```python
from build123d import *

# Parameters (mm, degrees)
PAD001_DEPTH        = 35
HOLE002_D           = 5.5
HOLE002_CSINK_D     = 10
HOLE002_CSINK_ANGLE = 90
SKETCH004_R         = 6.501169
SKETCH004_R_2       = 5.481256
POCKET_DEPTH        = 13.6312167212
SKETCH007_W         = 3.5
SKETCH007_H         = 35
POCKET002_DEPTH     = 1
CHAMFER_SIZE        = 0.99
FILLET007_R         = 3
FILLET008_R         = 1


with BuildPart() as part:
    # Sketch002 → Pad001 (new body)
    with BuildSketch(Plane.YZ):
        with BuildLine():
            Line((-188.1964293023, 612.8903873712), (-179.4587343049, 634.2262558534))
            Line((-171.1300961638, 630.8154221261), (-179.4587343049, 634.2262558534))
            Line((-169.4299601233, 597.7008988779), (-171.1300961638, 630.8154221261))
            Line((-173.2197753758, 588.446856499), (-169.4299601233, 597.7008988779))
            Line((-191.7278601338, 596.0264870041), (-173.2197753758, 588.446856499))
            ThreePointArc((-191.7278601338, 596.0264870041), (-183.7026179221, 603.1476439882), (-188.1964293023, 612.8903873712))
        make_face()
    extrude(amount=PAD001_DEPTH)

    # Hole002 (through all)
    with Locations(Plane(origin=(0, -364.0835541104, 149.1034242189), x_dir=(0, 0.3789815253, 0.9254042379), z_dir=(0, 0.9254042379, -0.3789815253))):
        with Locations((-506.967621, 13.13074), (501.9041201044, 17.5)):
            CounterSinkHole(HOLE002_D / 2, HOLE002_CSINK_D / 2, counter_sink_angle=HOLE002_CSINK_ANGLE)

    # Sketch004 (on DatumPlane) → Pocket (cut, through all)
    with BuildSketch(Plane(origin=(0, -364.0835541104, 149.1034242189), x_dir=(0, 0.3789815253, 0.9254042379), z_dir=(0, 0.9254042379, -0.3789815253))):
        with Locations((-506.967621, 13.13074)):
            Circle(SKETCH004_R)
        with Locations((501.9041201044, 17.5)):
            Circle(SKETCH004_R_2)
    extrude(amount=POCKET_DEPTH, mode=Mode.SUBTRACT)

    # Sketch007 (on Face6 of Pocket) → Pocket002 (cut)
    with BuildSketch(Plane(origin=(0, -376.1138092031, 154.0301840472), x_dir=(0, -0.3789815253, -0.9254042379), z_dir=(0, -0.9254042379, 0.3789815253))):
        with Locations((-513.9041201044, 17.5)):
            Rectangle(SKETCH007_W, SKETCH007_H)
    extrude(amount=-POCKET002_DEPTH, mode=Mode.SUBTRACT)

    # Chamfer
    chamfer_edges = [part.edges().sort_by_distance(p)[0] for p in [
        (17.5, -179.76502, 630.839711),
        (17.5, -181.091455, 627.600796),
    ]]
    chamfer(chamfer_edges, length=CHAMFER_SIZE)

    # Fillet007
    fillet007_edges = [part.edges().sort_by_distance(p)[0] for p in [
        (17.5, -173.219775, 588.446856),
        (17.5, -188.196429, 612.890387),
        (17.5, -169.42996, 597.700899),
        (17.5, -171.130096, 630.815422),
        (17.5, -179.458734, 634.226256),
    ]]
    fillet(fillet007_edges, radius=FILLET007_R)

    # Fillet008
    fillet008_edges = [part.edges().sort_by_distance(p)[0] for p in [
        (17.5, -191.72786, 596.026487),
    ]]
    fillet(fillet008_edges, radius=FILLET008_R)


solid = part.part
```
Geometry check sheet. Reference: the model listing, model coordinates, mm. A direction names the side the tool comes from. Coordinates: 2 decimals unless noted, no trailing zeros. Loops run counter-clockwise (first coordinate to the right, second up) from the corner with the lowest first, then second, coordinate; pieces in that order, holes last. Notation, with made-up numbers: (37, -39) -> (41, -39) arc R22 cw to (41, -14) -> close; hole circle Ø3 at (55, 84). An arc over 180 degrees is marked (long way). Put each result on its own line as item: value.
1) Gauge pin test, flat ends, axial feed: pin 1 Ø12 at (x, y) = (18, -182) entering from +Z; pin 2 Ø2 at (x, y) = (9, -183.5) entering from -Z; pin 3 Ø6 at (x, y) = (26.5, -183.5) entering from +Z; pin 4 Ø4 at (x, z) = (28.5, 628) entering from -Y. Record the tip position at first contact, or that the pin passes through.
Result set:
pin 1: stops at z = 633.31
pin 2: stops at z = 592.25
pin 3: stops at z = 631.66
pin 4: stops at y = -182.83
2) Cross-section at B-B on z = 596. Record the boundary of the cut face in (x, y), plus the area to 3 significant figures.
Result set:
outline: (0, -189.54) -> (35, -189.54) -> (35, -170.13) -> (0, -170.13) -> close
area: 679 mm^2
3) Tool access check on faces 1 (the flat face through (17.745, -180.424, 629.23)), 2 (the cylindrical face through (17.745, -173.67, 589.606)). Record the directions out of +Z, -Z, +X, -X, +Y, -Y that give a thin tool (end or side, any length) a straight path to the whole face; none if there is none.
Result set:
face 1: +X, -X, -Y
face 2: -Z, +X, -X
4) Thickness scan on line 1 (Z direction, x = 19.5, y = -184.25); line 2 (X direction, y = -183.5, z = 618.5); line 3 (Z direction, x = 26, y = -185.25). Record the ranges inside material, lowest first.
Result set:
line 1: z = 592.96 to 601.42, 608.56 to 615.78, 619.86 to 622.53
line 2: x = 0 to 14.91, 20.09 to 35
line 3: z = 593.37 to 599.68, 610.31 to 620.09
5) Cross-section at C-C on z = 627. Record the boundary of the cut face in (x, y), plus the area to 3 significant figures.
Result set:
outline: (0, -182.42) -> (35, -182.42) -> (35, -170.93) -> (0, -170.93) -> close
area: 402 mm^2
6) Release check for a two-part mould opening along X. For faces 3 (the flat face through (35, -177, 612)), 4 (the cylindrical face through (17.745, -179.009, 633.067)), 5 (the cylindrical face through (18.33, -181.99, 614.06)), 6 (the cylindrical face through (17.74, -173.58, 607.53)) record: released by +X, released by -X, zero draft, split by the parting line, or undercut.
Result set:
face 3: released by +X
face 4: zero draft
face 5: undercut
face 6: undercut
